```python
from build123d import *


# Read off the part's stored shape, not the designer's step: M3x0.5 Tapped Hole1
with BuildPart() as part:
    # Sketch1 → Revolve1 (revolve)
    with BuildSketch(Plane(origin=(0, 0, 0), x_dir=(0, 0, -1), z_dir=(1, 0, 0)), mode=Mode.PRIVATE) as revolve1_sk:
        with BuildLine():
            Line((111.125, 0), (111.125, 2.9718))
            Line((111.125, 2.9718), (94.9452, 2.9718))
            Line((94.9452, 2.9718), (94.9452, 9.9441))
            Line((94.9452, 9.9441), (91.9988, 9.9441))
            Line((91.9988, 9.9441), (91.9988, 14.732))
            ThreePointArc((91.9988, 14.732), (91.626825612, 15.630025612), (90.7288, 16.002))
            Line((90.7288, 16.002), (56.8452, 16.002))
            Line((56.8452, 16.002), (56.8452, 16.5989))
            ThreePointArc((56.8452, 16.5989), (56.473225612, 17.496925612), (55.5752, 17.8689))
            Line((55.5752, 17.8689), (0, 17.8689))
            Line((0, 17.8689), (0, 8.0137))
            Line((0, 8.0137), (-2.286, 8.0137))
            Line((-2.286, 8.0137), (-2.286, 1.5621))
            Line((-2.286, 1.5621), (-3.5814, 1.5621))
            Line((-3.5814, 1.5621), (-3.5814, 0))
            Line((-3.5814, 0), (111.125, 0))
        make_face()
    revolve(revolve1_sk.sketch.rotate(Axis((0, 0, 3.5814), (0, 0, -1)), 90), axis=Axis((0, 0, 3.5814), (0, 0, -1)))

    # M3x0.5 Tapped Hole1 outline → M3x0.5 Tapped Hole1 (revolve, cut)
    with BuildSketch(Plane(origin=(-9, -9, 0), x_dir=(1, 0, 0), z_dir=(0, -1, 0))):
        Polygon((1.25, -86.9188), (0, -86.167724226), (0, -91.9988), (1.25, -91.9988), align=None)
    revolve(axis=Axis((-9, -9, 0), (0, 0, 1)), mode=Mode.SUBTRACT)

    # M3x0.5 Tapped Hole1 2 outline → M3x0.5 Tapped Hole1 2 (revolve, cut)
    with BuildSketch(Plane(origin=(9, 9, 0), x_dir=(1, 0, 0), z_dir=(0, -1, 0))):
        Polygon((1.25, -86.9188), (0, -86.167724226), (0, -91.9988), (1.25, -91.9988), align=None)
    revolve(axis=Axis((9, 9, 0), (0, 0, 1)), mode=Mode.SUBTRACT)

    # M3x0.5 Tapped Hole1 3 outline → M3x0.5 Tapped Hole1 3 (revolve, cut)
    with BuildSketch(Plane(origin=(9, -9, 0), x_dir=(1, 0, 0), z_dir=(0, -1, 0))):
        Polygon((1.25, -86.9188), (0, -86.167724226), (0, -91.9988), (1.25, -91.9988), align=None)
    revolve(axis=Axis((9, -9, 0), (0, 0, 1)), mode=Mode.SUBTRACT)

    # M3x0.5 Tapped Hole1 4 outline → M3x0.5 Tapped Hole1 4 (revolve, cut)
    with BuildSketch(Plane(origin=(-9, 9, 0), x_dir=(1, 0, 0), z_dir=(0, -1, 0))):
        Polygon((1.25, -86.9188), (0, -86.167724226), (0, -91.9988), (1.25, -91.9988), align=None)
    revolve(axis=Axis((-9, 9, 0), (0, 0, 1)), mode=Mode.SUBTRACT)


solid = part.part
```
The listing builds one solid part. Answer for the finished solid, in the listing's coordinates (mm). A direction names the side the tool comes from. Give positions to 0.01 mm unless a question says otherwise; leave off trailing zeros. Write each loop counter-clockwise with the first axis right and the second up, starting at its lowest first coordinate (ties: lowest second). Pieces come first, ordered by that corner, then holes. Notation, with made-up numbers: (-30.75, 7.5) -> (11.25, 7.5) arc R16 cw to (11.25, 27.5) -> close; hole circle Ø5 at (73, 83). An arc over 180 degrees is marked (long way). Use one line per item in the form item = value.
1) Section B-B on z = -62.5 is taken. Write down the section's boundary in (x, y), plus the area to 3 significant figures.
Result:
outline = circle Ø32 at (0, 0)
area = 804 mm²
2) Section C-C on z = -32.5 is taken. Write down the section's boundary in (x, y), plus the area to 3 significant figures.
Result:
outline = circle Ø35.74 at (0, 0)
area = 1,000 mm²
3) Straight lines are drawn through the part: probe 1 along Y at (x, z) = (-9, -88.8); probe 2 along Z at (x, y) = (-8.5, -12); probe 3 along X at (y, z) = (-0.5, -76). For each, find the intervals that lie inside material, in ascending order.
Result:
probe_1 = -13.23 to -10.25, -7.75 to 7.75, 10.25 to 13.23
probe_2 = -92 to 0
probe_3 = -15.99 to 15.99
4) Each of these flat-tipped pins is pushed along its axis until it touches: P1, Ø12, axis at x = -14, y = 6, coming from the +Z side; P2, Ø6, axis at x = 11, z = -21, coming from the +Y side; P3, Ø1.5, axis at x = -5.5, z = -18, coming from the -Y side. Where does it stop, or does it pass through?
Result:
P1 = 0
P2 = 15.98
P3 = -17.23
5) A tool of negligible diameter and unlimited length cuts with its end or side. For faces 1 (the cylindrical face through (-9.921, 9.845, -89.423)), 2 (the cylindrical face through (1.49, -0.47, 2.94)), 3 (the flat face through (0, 0, -111.125)), from which of +Z, -Z, +X, -X, +Y, -Y can it reach the whole face along a straight path? Write none if from no direction.
Result:
face_1 = -Z
face_2 = +Z
face_3 = -Z, +X, -X, +Y, -Y
6) For a pull along Y with two mould halves and no side action, classify faces 4 (the cylindrical face through (-3.874, 17.444, -27.399)), 5 (the conical face through (-9.2, -8.99, -86.29)), 6 (the flat face through (4, 8, 0)) as +Y half, -Y half, draft (parallel to the pull), parting line (faces both ways), or undercut.
Result:
face_4 = parting line
face_5 = undercut
face_6 = draft
7) Section A-A on x = 0 is taken. Write down the section's boundary in (y, z) (3 decimals).
Result:
outline = (-17.869, -55.575) arc R1.27 ccw to (-16.599, -56.845) -> (-16.002, -56.845) -> (-16.002, -90.729) arc R1.27 ccw to (-14.732, -91.999) -> (-9.944, -91.999) -> (-9.944, -94.945) -> (-2.972, -94.945) -> (-2.972, -111.125) -> (2.972, -111.125) -> (2.972, -94.945) -> (9.944, -94.945) -> (9.944, -91.999) -> (14.732, -91.999) arc R1.27 ccw to (16.002, -90.729) -> (16.002, -56.845) -> (16.599, -56.845) arc R1.27 ccw to (17.869, -55.575) -> (17.869, 0) -> (8.014, 0) -> (8.014, 2.286) -> (1.562, 2.286) -> (1.562, 3.581) -> (-1.562, 3.581) -> (-1.562, 2.286) -> (-8.014, 2.286) -> (-8.014, 0) -> (-17.869, 0) -> close
